Design review of the part shown in the three views and the two pictorial views. Dimensions are in mm from the part's minimum x, y and z. Round coordinates to 2 decimals unless told otherwise and drop trailing zeros. Write each loop counter-clockwise with the first axis right and the second up, starting at its lowest first coordinate (ties: lowest second). Pieces come first, ordered by that corner, then holes. Notation, with made-up numbers: (36, 51) -> (80, 51) arc R21 ccw to (80, 83) -> close; hole circle Ø3 at (-9.5, 31.25). An arc over 180 degrees is marked (long way). Return JSON: item names as keys, results as strings. Group by question number.
1. For line 1 along Y through (x, z) = (82.5, 0.6) (3 decimals); line 2 along X through (y, z) = (119, 0.2), list the stretches that pass through material, from the lowest coordinate up. Write a range as from..to.
2. Take a section at B-B, the plane z = 2.2. Write out the cut boundary in (x, y) (3 decimals), then the cut area to 3 significant figures.
3. Clearance check with a flat-ended pin moving along its axis: P1, Ø8, axis at x = 70.5, y = 108, coming from the -Z side. State where the tip first meets the part, or that it passes through.
4. Take a section at C-C, the plane x = 18. Write out the cut boundary in (y, z) (3 decimals).
5. Take a section at A-A, the plane y = 119. Write out the cut boundary in (x, z) (3 decimals).
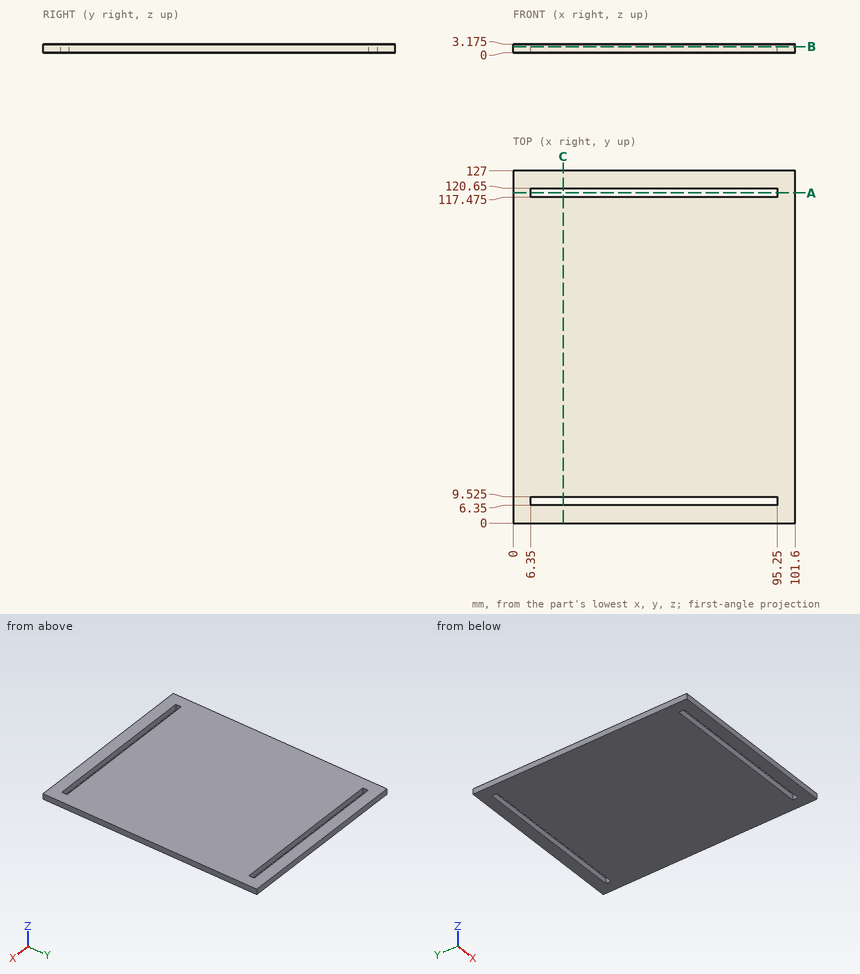
Output:
{
 "1": {"line 1": "y = 0..6.35, 9.525..117.475, 120.65..127", "line 2": "x = 0..6.35, 95.25..101.6"},
 "2": {"outline": "(0, 0) -> (101.6, 0) -> (101.6, 127) -> (0, 127) -> close; hole (6.35, 6.35) -> (95.25, 6.35) -> (95.25, 9.525) -> (6.35, 9.525) -> close; hole (6.35, 117.475) -> (95.25, 117.475) -> (95.25, 120.65) -> (6.35, 120.65) -> close", "area": "12,300 mm^2"},
 "3": {"P1": "stops at z = 0"},
 "4": {"outline": "(0, 0) -> (6.35, 0) -> (6.35, 3.175) -> (0, 3.175) -> close; (9.525, 0) -> (117.475, 0) -> (117.475, 3.175) -> (9.525, 3.175) -> close; (120.65, 0) -> (127, 0) -> (127, 3.175) -> (120.65, 3.175) -> close"},
 "5": {"outline": "(0, 0) -> (6.35, 0) -> (6.35, 3.175) -> (0, 3.175) -> close; (95.25, 0) -> (101.6, 0) -> (101.6, 3.175) -> (95.25, 3.175) -> close"}
}
